Input: part model. Units: mm. Frame: model coordinates. A direction names the side the tool comes from. Coordinates: 2 decimals unless noted, no trailing zeros. Write each loop counter-clockwise with the first axis right and the second up, starting at its lowest first coordinate (ties: lowest second). Pieces come first, ordered by that corner, then holes. Notation, with made-up numbers: (19, 45.25) -> (71, 45.25) arc R20 ccw to (71, 75.25) -> close; hole circle Ø11 at (-19, 28.25). An arc over 180 degrees is marked (long way). One line per question, with ' | ' between items. Start each with the question number.
Autodesk Inventor part; units mm, degrees
ref_plane "YZ Plane" through (0, 0, 0) normal (1, 0, 0) x (0, 1, 0)
ref_plane "XY Plane" through (0, 0, 0) normal (0, 0, 1) x (1, 0, 0)
ref_plane "Work Plane1" through (0, 1.5875, 0) normal (0, 1, 0) x (-1, 0, 0)
sketch "Sketch8" plane through (0, 0, 0) normal (0, 1, 0) x (-1, 0, 0)
  line L0 (0, 0) -> (22.225, 0)
  line L1 (22.225, 0) -> (22.225, -5.08)
  line L2 (22.225, -5.08) -> (3.175, -5.08)
  line L3 (3.175, -5.08) -> (3.175, -10.16)
  line L4 (3.175, -10.16) -> (22.225, -10.16)
  line L5 (22.225, -10.16) -> (22.225, -15.2317)
  line L6 (22.225, -15.2317) -> (3.175, -15.2317)
  line L7 (3.175, -15.2317) -> (3.175, -20.3117)
  line L8 (3.175, -20.3117) -> (22.225, -20.3117)
  line L9 (22.225, -20.3117) -> (22.225, -25.393)
  line L10 (22.225, -25.393) -> (0, -25.393)
  dimension "d24" = 22.225
  dimension "d25" = 5.08
  dimension "d26" = 19.05
  dimension "d27" = 5.08
  dimension "d28" = 5.08
sketch "Sketch9" plane through (0, 0, 0) normal (1, 0, 0) x (0, 1, 0)
  circle A0 centre (0, 0) radius 0.889
  dimension "d29" = 1.778
sketch "Sketch10" plane through (0, 1.5875, 0) normal (0, 1, 0) x (-1, 0, 0)
  line L0 (0, 2.9232) -> (25.4, 2.9232)
  line L1 (25.4, 2.9232) -> (25.4, -28.8268)
  line L2 (25.4, -28.8268) -> (0, -28.8268)
  line L3 (0, -28.8268) -> (0, 2.9232)
  point P0 (0, 0)
  dimension "d30" = 25.4
  dimension "d32" = 31.75
extrude "Extrusion4" add sketch "Sketch10" against normal blind 3.175
sweep "Sweep2" cut profiles "Sketch9" path "Sketch8"
properties part number "strain gauge v2"
1) First-contact query: P1, Ø1.4, axis at y = 0, z = -5.08, coming from the +X side. Flat tip, straight axial feed; report the tip coordinate or a pass-through.
2) Section B-B, the plane x = -21.75. Return loops of the section in (y, z) (1 decimal), then the cut area to 3 significant figures.
3) Section A-A, the plane y = 0. Return loops of the section in (x, z).
4) Ray query, line 1 (Y direction, x = -12.75, z = 0); line 2 (X direction, y = 0, z = -22.5); line 3 (Y direction, x = -9.25, z = -25). Return the intervals inside material, ascending.
5) Section D-D, the plane z = -10.5. Return loops of the section in (x, y) (1 decimal), then the cut area to 3 significant figures.
6) Pull-direction query (Z, two-part tool) for faces 4 (the face through (-13, 0, 2.923)), 5 (the face through (0, 0, -13)), 6 (the face through (-13, 0, -28.827)), 7 (the face through (-2.294, -0.116, -17.82)); classes: released by +Z, released by -Z, zero draft, split by the parting line, or undercut.
7) Access query for faces 1 (the face through (-11.72, -0.19, 0.87)), 2 (the face through (-13, -1.588, -13)), 3 (the face through (-12.55, -0.12, -14.35)). Directions: +Z, -Z, +X, -X, +Y, -Y. A direction counts if a zero-diameter tool reaches every point of the face in a straight line with its end or side. Return the directions, or none.
8) Section C-C, the plane x = -7.25. Return loops of the section in (y, z), then the cut area to 3 significant figures.
Answer block:
1) P1: stops at x = 0
2) outline: (-1.6, -28.8) -> (1.6, -28.8) -> (1.6, 2.9) -> (-1.6, 2.9) -> close; hole (-0.8, -24.9) arc R0.9 ccw (long way) to (0.8, -24.9) -> (0.8, -20.8) arc R0.9 ccw (long way) to (-0.8, -20.8) -> close; hole (-0.8, -14.8) arc R0.9 ccw (long way) to (0.8, -14.8) -> (0.8, -10.6) arc R0.9 ccw (long way) to (-0.8, -10.6) -> close; hole (-0.8, -4.6) arc R0.9 ccw (long way) to (0.8, -4.6) -> (0.8, -0.5) arc R0.9 ccw (long way) to (-0.8, -0.5) -> close | area: 69.9 mm2
3) outline: (-25.4, -28.83) -> (0, -28.83) -> (0, -26.28) -> (-23.11, -26.28) -> (-23.11, -19.42) -> (-4.06, -19.42) -> (-4.06, -16.12) -> (-23.11, -16.12) -> (-23.11, -9.27) -> (-4.06, -9.27) -> (-4.06, -5.97) -> (-23.11, -5.97) -> (-23.11, 0.89) -> (0, 0.89) -> (0, 2.92) -> (-25.4, 2.92) -> close; (-21.34, -24.5) -> (0, -24.5) -> (0, -0.89) -> (-21.34, -0.89) -> (-21.34, -4.19) -> (-2.29, -4.19) -> (-2.29, -11.05) -> (-21.34, -11.05) -> (-21.34, -14.34) -> (-2.29, -14.34) -> (-2.29, -21.2) -> (-21.34, -21.2) -> close
4) line 1: y = -1.59 to -0.89, 0.89 to 1.59 | line 2: x = -25.4 to -23.11, -21.34 to 0 | line 3: y = -1.59 to -0.8, 0.8 to 1.59
5) outline: (-25.4, -1.6) -> (0, -1.6) -> (0, 1.6) -> (-25.4, 1.6) -> close; hole (-21.9, -0.8) -> (-2.8, -0.8) arc R0.9 ccw to (-2.8, 0.8) -> (-21.9, 0.8) arc R0.9 ccw (long way) to start | area: 46.9 mm2
6) face 4: released by +Z | face 5: zero draft | face 6: released by -Z | face 7: undercut
7) face 1: +X | face 2: +Z, -Z, +X, -X, -Y | face 3: none
8) outline: (-1.59, -28.83) -> (1.59, -28.83) -> (1.59, 2.92) -> (-1.59, 2.92) -> close; hole circle Ø1.78 at (0, -25.39); hole circle Ø1.78 at (0, -20.31); hole circle Ø1.78 at (0, -15.23); hole circle Ø1.78 at (0, -10.16); hole circle Ø1.78 at (0, -5.08); hole circle Ø1.78 at (0, 0) | area: 85.9 mm2
